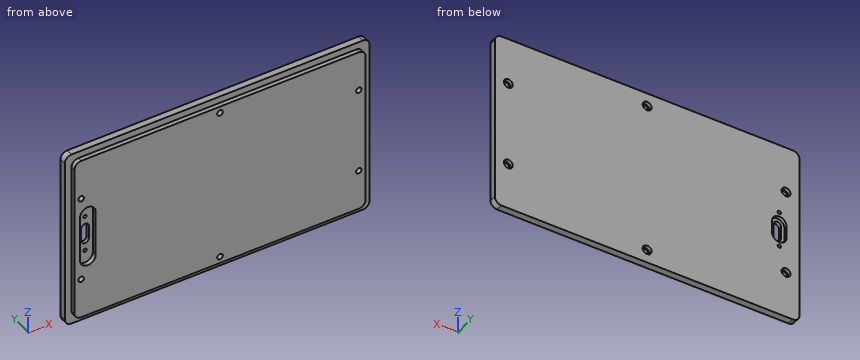
```python
from build123d import *

# Parameters (mm, degrees)
BOSS_EXTRUDE2_DEPTH      = 3
BOSS_EXTRUDE3_DEPTH      = 2
BOSS_EXTRUDE3_DEPTH_BACK = 3
CUT_EXTRUDE1_DEPTH       = 80.000063291
CUT_EXTRUDE1_DEPTH_BACK  = 80.000063291
SKETCH8_R                = 1.25
SKETCH9_W                = 7
SKETCH9_H                = 20.5
CUT_EXTRUDE2_DEPTH       = 2
SKETCH10_R               = 0.75
CUT_EXTRUDE3_DEPTH       = 80.000063291
SKETCH11_R               = 3.5
CUT_EXTRUDE4_DEPTH       = 2
SKETCH12_R               = 1.25
CUT_EXTRUDE6_DEPTH       = 80.101264212
CUT_EXTRUDE7_DEPTH       = 1.5
SKETCH19_R               = 2
CUT_EXTRUDE9_DEPTH       = 1.5


with BuildPart() as part:
    # Sketch1 → Boss-Extrude2 (new body)
    with BuildSketch(Plane(origin=(0, 0, 0), x_dir=(1, 0, 0), z_dir=(0, 1, 0))):
        with BuildLine():
            Line((65, 40.1), (-65, 40.1))
            ThreePointArc((-65, 40.1), (-67.121320344, 39.221320344), (-68, 37.1))
            Line((-68, 37.1), (-68, -37.1))
            ThreePointArc((-68, -37.1), (-67.121320344, -39.221320344), (-65, -40.1))
            Line((-65, -40.1), (65, -40.1))
            ThreePointArc((65, -40.1), (67.121320344, -39.221320344), (68, -37.1))
            Line((68, -37.1), (68, 37.1))
            ThreePointArc((68, 37.1), (67.121320344, 39.221320344), (65, 40.1))
        make_face()
        with BuildLine():
            Line((65, -34.1), (65, 34.1))
            ThreePointArc((65, 34.1), (64.121320344, 36.221320344), (62, 37.1))
            Line((62, 37.1), (-62, 37.1))
            ThreePointArc((-62, 37.1), (-64.121320344, 36.221320344), (-65, 34.1))
            Line((-65, 34.1), (-65, -34.1))
            ThreePointArc((-65, -34.1), (-64.121320344, -36.221320344), (-62, -37.1))
            Line((-62, -37.1), (62, -37.1))
            ThreePointArc((62, -37.1), (64.121320344, -36.221320344), (65, -34.1))
        make_face(mode=Mode.SUBTRACT)
    extrude(amount=BOSS_EXTRUDE2_DEPTH)

    # Sketch7 → Boss-Extrude3 (add, two sides: drawn at the far end of the back side and taken through both)
    with BuildSketch(Plane.XZ.offset(-BOSS_EXTRUDE3_DEPTH_BACK)):
        with BuildLine():
            Line((-62, 37.1), (62, 37.1))
            ThreePointArc((62, 37.1), (64.121320344, 36.221320344), (65, 34.1))
            Line((65, 34.1), (65, -34.1))
            ThreePointArc((65, -34.1), (64.121320344, -36.221320344), (62, -37.1))
            Line((62, -37.1), (-62, -37.1))
            ThreePointArc((-62, -37.1), (-64.121320344, -36.221320344), (-65, -34.1))
            Line((-65, -34.1), (-65, 34.1))
            ThreePointArc((-65, 34.1), (-64.121320344, 36.221320344), (-62, 37.1))
        make_face()
    extrude(amount=BOSS_EXTRUDE3_DEPTH + BOSS_EXTRUDE3_DEPTH_BACK)

    # Sketch8 → Cut-Extrude1 (cut, two sides: drawn at the far end of the back side and taken through both)
    with BuildSketch(Plane(origin=(0, 0, 0), x_dir=(1, 0, 0), z_dir=(0, 1, 0)).offset(-CUT_EXTRUDE1_DEPTH_BACK)):
        with Locations(Location((62, 19.1, 0), (0, 0, 90))):
            Circle(SKETCH8_R)
        with Locations(Location((62, -19.1, 0), (0, 0, 90))):
            Circle(SKETCH8_R)
        with Locations(Location((-62, -19.1, 0), (0, 0, 270))):
            Circle(SKETCH8_R)
        with Locations(Location((-62, 19.1, 0), (0, 0, 270))):
            Circle(SKETCH8_R)
    extrude(amount=CUT_EXTRUDE1_DEPTH + CUT_EXTRUDE1_DEPTH_BACK, mode=Mode.SUBTRACT)

    # Sketch9 → Cut-Extrude2 (cut)
    with BuildSketch(Plane.XZ.offset(2)):
        with Locations((-59, 0.15)):
            Rectangle(SKETCH9_W, SKETCH9_H)
    extrude(amount=-CUT_EXTRUDE2_DEPTH, mode=Mode.SUBTRACT)

    # Sketch10 → Cut-Extrude3 (cut, through all)
    with BuildSketch(Plane.XZ):
        with Locations(Location((-59, -7.85, 0), (0, 0, 270))):
            Circle(SKETCH10_R)
        with Locations(Location((-59, 8.15, 0), (0, 0, 270))):
            Circle(SKETCH10_R)
        with BuildLine():
            Line((-60.7, -2.75), (-60.7, 3.05))
            ThreePointArc((-60.7, 3.05), (-59, 4.75), (-57.3, 3.05))
            Line((-57.3, 3.05), (-57.3, -2.75))
            ThreePointArc((-57.3, -2.75), (-59, -4.45), (-60.7, -2.75))
        make_face()
    extrude(amount=-CUT_EXTRUDE3_DEPTH, mode=Mode.SUBTRACT)

    # Sketch11 → Cut-Extrude4 (cut)
    with BuildSketch(Plane.XZ.offset(2)):
        with Locations((-59, 10.4)):
            Circle(SKETCH11_R)
        with Locations((-59, -10.1)):
            Circle(SKETCH11_R)
    extrude(amount=-CUT_EXTRUDE4_DEPTH, mode=Mode.SUBTRACT)

    # Sketch12 → Cut-Extrude6 (cut, through all)
    with BuildSketch(Plane.XZ.offset(2)):
        with Locations(Location((0, -34.1, 0), (0, 0, 270))):
            Circle(SKETCH12_R)
        with Locations(Location((0, 34.1, 0), (0, 0, 270))):
            Circle(SKETCH12_R)
    extrude(amount=-CUT_EXTRUDE6_DEPTH, mode=Mode.SUBTRACT)

    # Sketch14 → Cut-Extrude7 (cut)
    with BuildSketch(Plane(origin=(0, 3, 0), x_dir=(1, 0, 0), z_dir=(0, 1, 0))):
        with BuildLine():
            Line((-62.2, 2.75), (-62.2, -3.05))
            ThreePointArc((-62.2, -3.05), (-59, -6.25), (-55.8, -3.05))
            Line((-55.8, -3.05), (-55.8, 2.75))
            ThreePointArc((-55.8, 2.75), (-59, 5.95), (-62.2, 2.75))
        make_face()
    extrude(amount=-CUT_EXTRUDE7_DEPTH, mode=Mode.SUBTRACT)

    # Sketch19 → Cut-Extrude9 (cut)
    with BuildSketch(Plane(origin=(0, 3, 0), x_dir=(1, 0, 0), z_dir=(0, 1, 0))):
        with Locations(Location((-62, -19.1, 0), (0, 0, 270))):
            Circle(SKETCH19_R)
        with Locations(Location((-62, 19.1, 0), (0, 0, 270))):
            Circle(SKETCH19_R)
        with Locations(Location((0, 34.1, 0), (0, 0, 270))):
            Circle(SKETCH19_R)
        with Locations(Location((0, -34.1, 0), (0, 0, 270))):
            Circle(SKETCH19_R)
        with Locations(Location((62, -19.1, 0), (0, 0, 270))):
            Circle(SKETCH19_R)
        with Locations(Location((62, 19.1, 0), (0, 0, 270))):
            Circle(SKETCH19_R)
    extrude(amount=-CUT_EXTRUDE9_DEPTH, mode=Mode.SUBTRACT)


solid = part.part
```
Model file for the job. Use its own axes, mm. Round coordinates to 2 decimals unless told otherwise and drop trailing zeros. Loops run counter-clockwise (first coordinate to the right, second up) from the corner with the lowest first, then second, coordinate; pieces in that order, holes last. Notation, with made-up numbers: M -23,-32.75 L 22,-32.75 A11 ccw 22,-28.75 Z; hole C -39.5,-34 d8. An arc over 180 degrees is marked long. Put each result on its own line as item: value. Start each with the question number.
Item 1: Cut at C-C (x = -39). List the corners of the cut face in (y, z), then the cut area to 3 significant figures.
Item 2: Drill centre lines: line 1 along X through (y, z) = (0.55, 19.1); line 2 along X through (y, z) = (2.35, 19.1); line 3 along X through (y, z) = (2, -1.5). Where is each one in solid material? Low to high.
Item 3: Cut at B-B (z = -26). List the corners of the cut face in (x, y), then the cut area to 3 significant figures.
Item 4: Drop flat-ended pins along their axis: P1, Ø1, axis at y = -1.5, z = -2, coming from the -X side; P2, Ø3, axis at x = 62, z = -19.1, coming from the +Y side. Give the stop position or say it passes through.
Item 5: Cut at A-A (y = -1.2). List the corners of the cut face in (x, z), then the cut area to 3 significant figures.
Answer block:
1. outline: M -2,-37.1 L 0,-37.1 L 0,-40.1 L 3,-40.1 L 3,40.1 L 0,40.1 L 0,37.1 L -2,37.1 Z
1. area: 389 mm2
2. line 1: -68 to -63.25, -60.75 to 60.75, 63.25 to 68
2. line 2: -68 to -64, -60 to 60, 64 to 68
2. line 3: -68 to -62.2, -55.8 to 68
3. outline: M -68,0 L -65,0 L -65,-2 L 65,-2 L 65,0 L 68,0 L 68,3 L -68,3 Z
3. area: 668 mm2
4. P1: x = -65
4. P2: y = 1.5
5. outline: M -65,-34.1 A3 ccw -62,-37.1 L 62,-37.1 A3 ccw 65,-34.1 L 65,34.1 A3 ccw 62,37.1 L -62,37.1 A3 ccw -65,34.1 Z; hole C -62,-19.1 d2.5; hole C -62,19.1 d2.5; hole M -62.5,-10.1 A3.5 ccw -55.5,-10.1 L -55.5,10.4 A3.5 ccw -62.5,10.4 Z; hole C 0,-34.1 d2.5; hole C 0,34.1 d2.5; hole C 62,-19.1 d2.5; hole C 62,19.1 d2.5
5. area: 9,430 mm2
